from build123d import *

# Parameters (mm, degrees)
SKETCH007_R  = 4
PAD003_DEPTH = 31
SKETCH001_R  = 4
PAD004_DEPTH = 31
PAD006_DEPTH = 4
PAD001_DEPTH = 4
SKETCH_R     = 4.1
PAD_DEPTH    = 80


with BuildPart() as rodhole01:
    # Sketch007 → Pad003 (new body)
    with BuildSketch(Plane.XZ.offset(16)):
        with Locations((3.5, 40)):
            Circle(SKETCH007_R)
    extrude(amount=-PAD003_DEPTH)


with BuildPart() as rodhole02:
    # Sketch001 → Pad004 (new body)
    with BuildSketch(Plane.YZ.offset(15.5)):
        with Locations((-3.5, 70)):
            Circle(SKETCH001_R)
        with Locations((-3.5, 10)):
            Circle(SKETCH001_R)
    extrude(amount=-PAD004_DEPTH)


with BuildPart() as obj1:
    # Sketch002 → Pad006 (new body)
    with BuildSketch(Plane.YZ.offset(-10)):
        Polygon((2.908588, 66.3), (2.908588, 73.7), (-3.5, 77.4), (-9.908588, 73.7), (-9.908588, 66.3), (-3.5, 62.6), align=None)
        Polygon((-3.5, 2.6), (2.908588, 6.3), (2.908588, 13.7), (-3.5, 17.4), (-9.908588, 13.7), (-9.908588, 6.3), align=None)
    extrude(amount=-PAD006_DEPTH)


with BuildPart() as cutblock:
    # Sketch008 → Pad001 (new body)
    with BuildSketch(Plane.XZ.offset(-9)):
        Polygon((9.908588, 36.3), (9.908588, 43.7), (3.5, 47.4), (-2.908588, 43.7), (-2.908588, 36.3), (3.5, 32.6), align=None)
    extrude(amount=-PAD001_DEPTH)

    # Fusion: union RodHole01, RodHole02, obj1
    add(rodhole01.part)
    add(rodhole02.part)
    add(obj1.part)


with BuildPart() as cut:
    # Sketch → Pad (new body)
    with BuildSketch(Plane.XY):
        with BuildLine():
            Line((-13.000011, 5.000021), (-13.000011, -13))
            Line((-13.000011, -13), (13.000011, -13))
            Line((13.000011, -13), (13.000011, 13))
            Line((13.000011, 13), (-5.00001, 13))
            ThreePointArc((-5.00001, 13), (-10.656858, 10.656862), (-13.000011, 5.000021))
        make_face()
        with Locations((-5.000011, 5)):
            Circle(SKETCH_R, mode=Mode.SUBTRACT)
    extrude(amount=PAD_DEPTH)

    # Cut: cut CutBlock
    add(cutblock.part, mode=Mode.SUBTRACT)


solid = cut.part
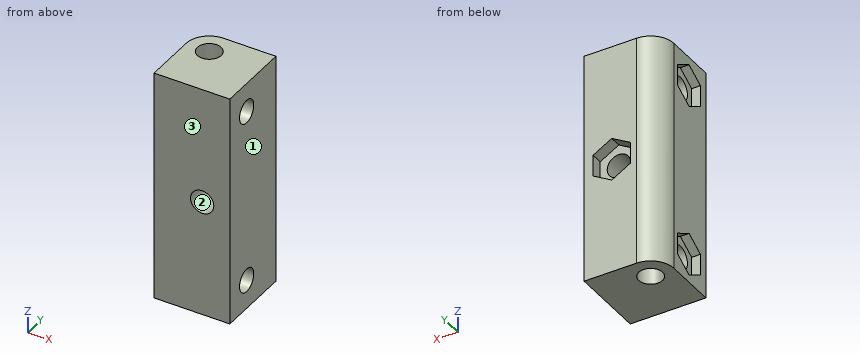
Source: CAD feature listing. Evaluate the final solid. Frame: model axes, mm. Face numbers are marked on the shaded views. Round coordinates to 2 decimals unless told otherwise and drop trailing zeros. Loops run counter-clockwise (first coordinate to the right, second up) from the corner with the lowest first, then second, coordinate; pieces in that order, holes last.
Q1. Section B-B, the plane y = -5.5. Return loops of the section in (x, z).
Q2. Ray query, line 1 (Z direction, x = -6.75, y = -2); line 2 (Z direction, x = -1.75, y = -3.5); line 3 (Z direction, x = 3.5, y = -8). Return the intervals inside material, ascending.
Q3. Section C-C, the plane x = -6. Return loops of the section in (y, z).
Q4. First-contact query: P1, Ø4.5, axis at y = 11.5, z = 38.5, coming from the -X side; P2, Ø6.5, axis at x = -5, y = 5, coming from the +Z side; P3, Ø2.5, axis at x = -12, z = 68.5, coming from the +Y side; P4, Ø0.9, axis at x = -12, z = 11, coming from the +Y side. Flat tips, straight axial feed; report the tip coordinate or a pass-through.
Q5. Mould query, pull axis X, two halves, no side actions, for the marked faces 1, 2 and 3. Classes: pulls with the +X half, pulls with the -X half, needs draft (parallel to the pull), parting line crosses it, or undercut.
Q6. Section D-D, the plane y = 6.5. Return loops of the section in (x, z).
Q7. Section A-A, the plane z = 70. Return loops of the section in (x, y).
Solutions:
1. outline: (-13, 0) - (13, 0) - (13, 6.54) - (-10, 6.54) - (-10, 3.75) - (-13, 3.75) - close; (-13, 16.25) - (-10, 16.25) - (-10, 13.46) - (13, 13.46) - (13, 66.54) - (-10, 66.54) - (-10, 63.75) - (-13, 63.75) - close; (-13, 76.25) - (-10, 76.25) - (-10, 73.46) - (13, 73.46) - (13, 80) - (-13, 80) - close; hole circle Ø8 at (3.5, 40)
2. line 1: z = 0 to 6.29, 13.71 to 66.29, 73.71 to 80
2. line 2: z = 0 to 6, 14 to 66, 74 to 80
2. line 3: z = 0 to 36, 44 to 80
3. outline: (-13, 0) - (1.02, 0) - (1.02, 80) - (-13, 80) - close; (8.98, 0) - (12.94, 0) - (12.94, 80) - (8.98, 80) - close; hole circle Ø8 at (-3.5, 10); hole circle Ø8 at (-3.5, 70)
4. P1: stops at x = -11.78
4. P2: passes through
4. P3: stops at y = 10.56
4. P4: stops at y = 9.59
5. face 1: pulls with the +X half
5. face 2: undercut
5. face 3: needs draft
6. outline: (-12.86, 0) - (-8.82, 0) - (-8.82, 80) - (-12.86, 80) - close; (-1.18, 0) - (13, 0) - (13, 80) - (-1.18, 80) - close; hole circle Ø8 at (3.5, 40)
7. outline: (-13, -13) - (13, -13) - (13, -7.5) - (-10, -7.5) - (-10, -9.91) - (-13, -9.91) - close; (-13, 2.91) - (-10, 2.91) - (-10, 0.5) - (13, 0.5) - (13, 13) - (-5, 13) arc R8 ccw to (-13, 5) - close; hole circle Ø8.2 at (-5, 5)
